Geometry check sheet. Reference: the model listing, model coordinates, mm. Face numbers are marked on the shaded views. A direction names the side the tool comes from. Give positions to 0.01 mm unless a question says otherwise; leave off trailing zeros. Write each loop counter-clockwise with the first axis right and the second up, starting at its lowest first coordinate (ties: lowest second). Pieces come first, ordered by that corner, then holes. Notation, with made-up numbers: (-39, 77) - (1, 77) arc R15 cw to (1, 85) - close; hole circle Ø7 at (17, 16.5). An arc over 180 degrees is marked (long way). Write item = value, one per line. Start each with the question number.
(1) Depth check by flat-ended pin: pin 1 Ø1.5 at (x, z) = (1, -2) entering from +Y; pin 2 Ø3 at (x, y) = (-1.5, -2) entering from +Z; pin 3 Ø1 at (x, z) = (2, -1.5) entering from +Y. Enter the tip coordinate at first touch or a pass-through.
(2) Thickness scan on L1, parallel to X at y = 0.15, z = 0.5; L2, parallel to X at y = -0.8, z = 0.75; L3, parallel to Y at x = 0.5, z = 1.75. Record the ranges inside material, lowest first.
(3) Section check A-A, the plane z = 1.5. Enter the section's corners in (x, y).
(4) Access from +Z, -Z, +X, -X, +Y, -Y to the whole of each face (thin tool, end or side, straight path). Record for the marked faces 1, 2 and 3.
(5) Section check B-B, the plane y = -1.1. Enter the section's corners in (x, z), plus the area to 3 significant figures.
(6) Section check C-C, the plane z = 2.5. Enter the section's corners in (x, y).
```python
from build123d import *

# Parameters (mm, degrees)
F0_R          = 3
F1_DEPTH      = 1
F2_R          = 2.4
F2_R_2        = 1.4
F3_DEPTH      = 2
F4_W          = 2
F4_H          = 2
F5_DEPTH      = 2
F6_SIZE       = 1.5
F8_DEPTH      = 25
F8_DEPTH_BACK = 25
F11_DEPTH     = 25


with BuildPart() as f1:
    # F0 (on Front) → F1 (new body)
    with BuildSketch(Plane.XZ):
        Circle(F0_R)
    extrude(amount=F1_DEPTH)

    # F2 (on face) → F3 (join)
    with BuildSketch(Plane.XZ.offset(1)):
        Circle(F2_R)
        Circle(F2_R_2, mode=Mode.SUBTRACT)
        Circle(F2_R_2)
    extrude(amount=F3_DEPTH)

    # F4 (on face) → F5 (join)
    with BuildSketch(Plane(origin=(0, 0, 0), x_dir=(-1, 0, 0), z_dir=(0, 1, 0))):
        with Locations((0, 1)):
            Rectangle(F4_W, F4_H)
        with BuildLine():
            Line((-1, 0), (-3, 0))
            ThreePointArc((-3, 0), (0, -3), (3, 0))
            Line((3, 0), (1, 0))
            Line((1, 0), (-1, 0))
        make_face()
    extrude(amount=F5_DEPTH)

    # F6
    f6_edges = [f1.edges().sort_by_distance(p)[0] for p in [
        (0, 2, 2),
    ]]
    chamfer(f6_edges, length=F6_SIZE)

    # F7 (on face) → F8 (cut, two sides)
    with BuildSketch(Plane(origin=(-1, 0, 0), x_dir=(0, -1, 0), z_dir=(-1, 0, 0))) as f8_sk:
        with BuildLine():
            add(Edge.make_bspline(
                [(-2, 0.5), (-1.8012148761, 0.400607438), (-1.6024297521, 0.2238049575), (-1.4133396134, 0)],
                knots=[0, 0, 0, 0, 0.7803205861, 0.7803205861, 0.7803205861, 0.7803205861], degree=3))
            Line((-2, 0.5), (-2, 0))
            Line((-2, 0), (-1.4133396134, 0))
        make_face()
        with BuildLine():
            Line((-1.4133396134, 0), (-2, 0))
            Line((-2, 0), (-2, -3.0058792327))
            Line((-2, -3.0058792327), (-0.234228326, -3.0058792327))
            add(Edge.make_bspline(
                [(-1.4133396134, 0), (-0.651200933, -0.9020587545), (-0.0465611068, -2.5676912631), (-0.234228326, -3.0058792327)],
                knots=[0.7803205861, 0.7803205861, 0.7803205861, 0.7803205861, 3.9254475921, 3.9254475921, 3.9254475921, 3.9254475921], degree=3))
        make_face()
    extrude(amount=-F8_DEPTH, mode=Mode.SUBTRACT)
    extrude(f8_sk.sketch, amount=F8_DEPTH_BACK, mode=Mode.SUBTRACT)

    # F10 (on face) + F9 (on face) → F11 (cut)
    with BuildSketch(Plane.XY):
        Polygon((-2, 1.4133396134), (-3, 1.4133396134), (-3, 0.4133396134), align=None)
    with BuildSketch(Plane.XY):
        Polygon((3, 0.4133396134), (3, 1.4133396134), (2, 1.4133396134), align=None)
    extrude(amount=-F11_DEPTH, mode=Mode.SUBTRACT)


solid = f1.part
```
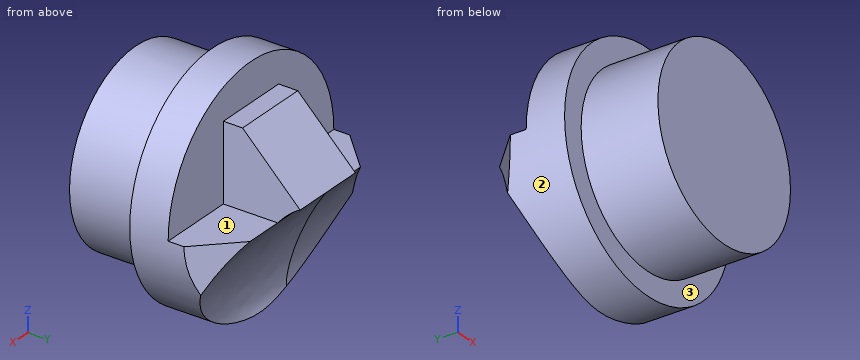
Model answer:
q1.pin_1 = 0.65
q1.pin_2 = 2.98
q1.pin_3 = 0.77
q2.L1 = -1 to 1
q2.L2 = -2.9 to 2.9
q2.L3 = -3 to 0.75
q3.outline = (-2.6, -1) - (-1.87, -1) - (-1.87, -3) - (1.87, -3) - (1.87, -1) - (2.6, -1) - (2.6, 0) - (1, 0) - (1, 1) - (-1, 1) - (-1, 0) - (-2.6, 0) - close
q4.face_1 = +Z, +X, +Y
q4.face_2 = +Y, -Y
q4.face_3 = -Y
q5.outline = circle Ø4.8 at (0, 0)
q5.area = 18.1 mm²
q6.outline = (-1.66, -1) - (1.66, -1) - (1.66, 0) - (-1.66, 0) - close
